For this review, take the finished solid that the model builds, in its own axes (mm). Face numbers are marked on the shaded views. A direction names the side the tool comes from. Round coordinates to 2 decimals unless told otherwise and drop trailing zeros. Order: outer loops, then holes, each group sorted by start corner. A loop starts at its lowest first (then second) coordinate and runs counter-clockwise, first axis right, second up.
Autodesk Inventor part; units mm, degrees
ref_plane "to_bearing_XY" through (0, 27, -6.5) normal (0, 0, 1) x (1, 0, 0)
ref_plane "to_bearing_YZ" through (0, 27, -6.5) normal (1, 0, 0) x (0, 1, 0)
ref_plane "to_bearing_ZX" through (0, 27, -6.5) normal (0, 1, 0) x (0, 0, 1)
sketch "Sketch_7" plane through (0, 0, 0) normal (0, 0, 1) x (1, 0, 0)
  line L0 (-19, 27) -> (-19, 0)
  line L1 (-19, 0) -> (19, 0)
  line L2 (19, 0) -> (19, 27)
  arc A0 (19, 27) -> (-19, 27) centre (0, 27) ccw
extrude "Extrusion1" add sketch "Sketch_7" against normal blind 15
sketch "Sketch_8" plane through (0, 0, 0) normal (1, 0, 0) x (0, 0, -1)
  line L0 (15, 27) -> (2, 27)
  line L1 (2, 27) -> (2, 42)
  line L2 (2, 42) -> (11, 42)
  line L3 (11, 42) -> (11, 42.7)
  line L4 (11, 42.7) -> (12.2, 42.7)
  line L5 (12.2, 42.7) -> (12.2, 42)
  line L6 (12.2, 42) -> (15, 42)
  line L7 (15, 42) -> (15, 27)
  line L8 (15, 27) -> (2, 27)
revolve "Revolution1" cut sketch "Sketch_8" angle 360 about axis through (0, 27, -15) along (0, 0, -1)
sketch "Sketch_1" plane through (0, 0, 0) normal (1, 0, 0) x (0, 0, -1)
  line L0 (15, 27) -> (0, 27)
  line L1 (0, 27) -> (0, 39)
  line L2 (0, 39) -> (15, 39)
  line L3 (15, 39) -> (15, 27)
  line L4 (15, 27) -> (0, 27)
revolve "Revolution2" cut sketch "Sketch_1" angle 360 about axis through (0, 27, -15) along (0, 0, -1)
sketch "Sketch4" plane through (0, 0, -15) normal (0, 0, -1) x (-1, 0, 0)
  point P0 (7, 7)
hole "Hole1" at (-7, 7, -15) direction (0, 0, 1) diameter 6 depth 15
pattern_linear "Rectangular Pattern1" count 2 spacing 14 along (1, 0, 0) of "Hole1"
ref_plane "to_bearing_XY" through (0, 27, -6.5) normal (0, 0, 1) x (1, 0, 0)
ref_plane "to_bearing_YZ" through (0, 27, -6.5) normal (1, 0, 0) x (0, 1, 0)
ref_plane "to_bearing_ZX" through (0, 27, -6.5) normal (0, 1, 0) x (0, 0, 1)
ref_plane "to_retaining_ring_XY" through (0, 27, -12.2) normal (0, 0, -1) x (1, 0, 0)
ref_plane "to_retaining_ring_YZ" through (0, 27, -12.2) normal (1, 0, 0) x (0, -1, 0)
ref_plane "to_retaining_ring_ZX" through (0, 27, -12.2) normal (0, -1, 0) x (0, 0, -1)
properties part number "SBGSMA6200ZZ-20_h"
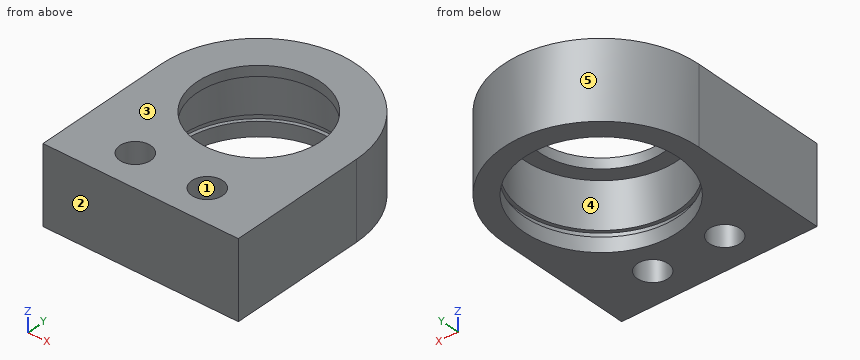
Q1. Wall thickness on line 1 (X direction, y = 7, z = -10.5); line 2 (X direction, y = 27, z = -9); line 3 (X direction, y = 27, z = -1.3): over which ranges is each line inside the solid? List them lowest first.
Q2. Take a section at B-B, the plane y = 7. State the section outline as (x, z) points, plus the area to 3 significant figures.
Q3. Take a section at A-A, the plane x = 0. State the section outline as (y, z) points, plus the area to 3 significant figures.
Q4. Clearance check with flat-ended pins moving along their axes: pin 1 (15.5 mm diameter, centred on x = 7, y = 26.5, fed in from -Z); pin 2 (3 mm diameter, centred on x = -13, z = -8.5, fed in from +Y); pin 3 (1.5 mm diameter, centred on x = -1.5, z = -2, fed in from +Y). State where each tip first meets the part, or that it passes through.
Q5. Take a section at C-C, the plane z = -11.5. State the section outline as (x, y) points.
Q6. Tool access review of the marked faces 4 and 5: name each direction out of +Z, -Z, +X, -X, +Y, -Y from which nothing blocks a thin tool from reaching the whole face with its end or side.
Q7. Take a section at D-D, the plane x = 7. State the section outline as (y, z) points, plus the area to 3 significant figures.
Q8. Mouldability with a two-part tool opening along Y and no side actions: class the marked faces 1, 2 and 3 as +Y half, -Y half, draft (parallel to the pull), parting line (faces both ways), or undercut.
Working result:
1. line 1: x = -19 to -10, -4 to 4, 10 to 19
1. line 2: x = -19 to -15, 15 to 19
1. line 3: x = -19 to -12, 12 to 19
2. outline: (-19, -15) - (-10, -15) - (-10, 0) - (-19, 0) - close; (-4, -15) - (4, -15) - (4, 0) - (-4, 0) - close; (10, -15) - (19, -15) - (19, 0) - (10, 0) - close
2. area: 390 mm2
3. outline: (0, -15) - (12, -15) - (12, -12.2) - (11.3, -12.2) - (11.3, -11) - (12, -11) - (12, -2) - (15, -2) - (15, 0) - (0, 0) - close; (39, -2) - (42, -2) - (42, -11) - (42.7, -11) - (42.7, -12.2) - (42, -12.2) - (42, -15) - (46, -15) - (46, 0) - (39, 0) - close
3. area: 250 mm2
4. pin 1: stops at z = -2
4. pin 2: stops at y = 42.12
4. pin 3: stops at y = 45.99
5. outline: (-19, 0) - (19, 0) - (19, 27) arc R19 ccw to (-19, 27) - close; hole circle Ø31.4 at (0, 27); hole circle Ø6 at (-7, 7); hole circle Ø6 at (7, 7)
6. face 4: -Z
6. face 5: +Z, -Z, +Y
7. outline: (0, -15) - (4, -15) - (4, 0) - (0, 0) - close; (10, -15) - (13.73, -15) - (13.73, -12.2) - (12.95, -12.2) - (12.95, -11) - (13.73, -11) - (13.73, -2) - (17.25, -2) - (17.25, 0) - (10, 0) - close; (36.75, -2) - (40.27, -2) - (40.27, -11) - (41.05, -11) - (41.05, -12.2) - (40.27, -12.2) - (40.27, -15) - (44.66, -15) - (44.66, 0) - (36.75, 0) - close
7. area: 194 mm2
8. face 1: undercut
8. face 2: -Y half
8. face 3: draft
